```python
from build123d import *

# Parameters (mm, degrees)
F0_W     = 23
F0_H     = 27
F0_W_2   = 22
F1_DEPTH = 3
F2_W     = 1.5
F2_H     = 1
F4_W     = 1.463154
F4_H     = 1.5


with BuildPart() as f1:
    # F0 (on Top) → F1 (new body)
    with BuildSketch(Plane.XY):
        Polygon((-59.5, 71.5), (-59.5, 24.5), (-47, 24.5), (-47, 29.5), (-29, 29.5), (-29, 24.5), (-19, 24.5), (-19, 27), (-2, 27), (-2, 24.5), (7, 24.5), (7, 29.5), (7.5, 29.5), (7.5, 34.5), (5.5, 34.5), (5.5, 61.5), (7.5, 61.5), (7.5, 71.5), align=None)
        with Locations((-38, 48)):
            Rectangle(F0_W, F0_H, mode=Mode.SUBTRACT)
        with Locations((-10.5, 48)):
            Rectangle(F0_W_2, F0_H, mode=Mode.SUBTRACT)
    extrude(amount=F1_DEPTH)

    # F2 (on face) → F3 (revolve)
    with BuildSketch(Plane.XZ.offset(-61.5)):
        with Locations((-37.25, 1.5)):
            Rectangle(F2_W, F2_H)
    revolve(axis=Axis((-38, 61.5, 1.5), (0, 0, -1)))

    # F4 (on face) → F5 (revolve)
    with BuildSketch(Plane.XZ.offset(-61.5)):
        with Locations((-11.231577, 2.25)):
            Rectangle(F4_W, F4_H)
        with Locations((-9.768423, 2.25)):
            Rectangle(F4_W, F4_H)
    revolve(axis=Axis((-10.5, 61.5, 1.5), (-1, 0, 0)))


solid = f1.part
```
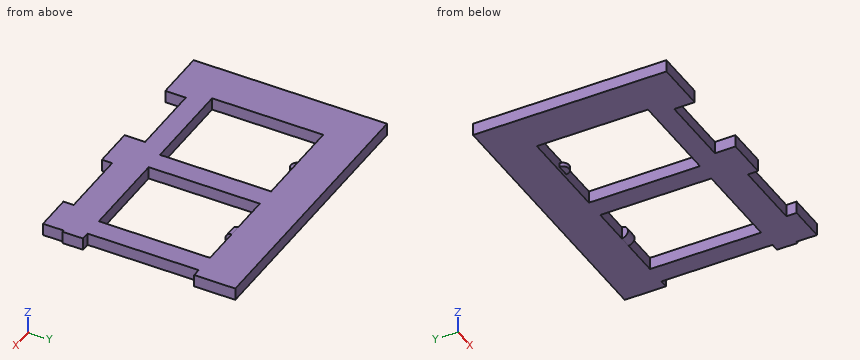
Work out the finished part from the listing and answer in its coordinate system (mm). Give positions to 0.01 mm unless a question says otherwise; leave off trailing zeros. Write each loop counter-clockwise with the first axis right and the second up, starting at its lowest first coordinate (ties: lowest second). Pieces come first, ordered by that corner, then holes.
(1) The part is cut by section D-D on x = -42. Write down the section's boundary in (y, z), plus the area to 3 significant figures.
Final values:
outline: (29.5, 0) - (34.5, 0) - (34.5, 3) - (29.5, 3) - close; (61.5, 0) - (71.5, 0) - (71.5, 3) - (61.5, 3) - close
area: 45.0 mm2
(2) Flat-ended cylindrical pins translate along their axes: pin 1 Ø1.6 at (x, y) = (-38, 60.5) entering from -Z; pin 2 Ø0.9 at (y, z) = (43.5, 2) entering from +X; pin 3 Ø1.2 at (x, y) = (-37.5, 60.5) entering from +Z. Find the tip coordinate at first contact, or state that the pin passes through.
Final values:
pin 1: stops at z = 1
pin 2: stops at x = 5.5
pin 3: stops at z = 2
(3) The part is cut by section A-A on x = -5. Write down the section's boundary in (y, z).
Final values:
outline: (27, 0) - (34.5, 0) - (34.5, 3) - (27, 3) - close; (61.5, 0) - (71.5, 0) - (71.5, 3) - (61.5, 3) - close
(4) The part is cut by section B-B on y = 55.5. Write down the section's boundary in (x, z).
Final values:
outline: (-59.5, 0) - (-49.5, 0) - (-49.5, 3) - (-59.5, 3) - close; (-26.5, 0) - (-21.5, 0) - (-21.5, 3) - (-26.5, 3) - close; (0.5, 0) - (5.5, 0) - (5.5, 3) - (0.5, 3) - close
(5) Straight lines are drawn through the part: line 1 (X direction, y = 35, z = 0.35); line 2 (X direction, y = 61, z = 2.45); line 3 (Y direction, x = -3.5, z = 1.3). For each, find the intervals that lie inside material, in ascending order.
Final values:
line 1: x = -59.5 to -49.5, -26.5 to -21.5, 0.5 to 5.5
line 2: x = -59.5 to -49.5, -26.5 to -21.5, -11.96 to -9.04, 0.5 to 5.5
line 3: y = 27 to 34.5, 61.5 to 71.5
(6) The part is cut by section C-C on z = 1.5. Count the separate pieces of the cut face and the enclosed holes in it, plus the area to 3 significant figures.
Final values:
separate pieces: 1
enclosed holes: 2
area: 1,750 mm2
